Verification items for the finished model (mm, model axes). A direction names the side the tool comes from. Coordinates: 2 decimals unless noted, no trailing zeros. Loops run counter-clockwise (first coordinate to the right, second up) from the corner with the lowest first, then second, coordinate; pieces in that order, holes last. Notation, with made-up numbers: (-30, -20) -> (15, -20) arc R21 cw to (15, 7) -> close; hole circle Ø8 at (-28.5, -22.75). An arc over 180 degrees is marked (long way). Answer as a JSON object with one key per item and string values. Group by question number.
Q1. Scan lines: L1, parallel to X at y = 15, z = 50; L2, parallel to X at y = 47, z = 15; L3, parallel to Z at x = 48, y = 44. Record each from-to range of solid material in increasing order.
Q2. Cross-section at C-C on x = 21. Record the boundary of the cut face in (y, z), and give its area (3 significant figures).
Q3. Gauge pin test, flat ends, axial feed: pin 1 Ø10 at (x, z) = (52, 52) entering from +Y; pin 2 Ø10 at (x, y) = (47.5, 46.5) entering from +Z; pin 3 Ø1 at (y, z) = (49, 13) entering from -X. Record the tip position at first contact, or that the pin passes through.
Q4. Set-up check for faces 1 (the flat face through (50, 50, 40)), 2 (the flat face through (10, 10, 20)), 3 (the flat face through (60, 30, 30)), 4 (the flat face through (40, 40, 24)): record each of +Z, -Z, +X, -X, +Y, -Y from which the full face is reachable in a straight line by a thin tool's end or side.
Q5. Cross-section at D-D on y = 55. Record the boundary of the cut face in (x, z).
Q6. Cross-section at A-A on z = 35.5. Record the boundary of the cut face in (x, y).
Q7. Cross-section at B-B on y = 5. Record the boundary of the cut face in (x, z).
```python
from build123d import *

# Parameters (mm, degrees)
ESBO_O1_W                = 60
ESBO_O1_H                = 20
RESSALTO_EXTRUS_O1_DEPTH = 20
ESBO_O2_W                = 40
ESBO_O2_H                = 20
RESSALTO_EXTRUS_O2_DEPTH = 40
ESBO_O3_W                = 20
ESBO_O3_H                = 60
RESSALTO_EXTRUS_O3_DEPTH = 20
ESBO_O4_W                = 20
ESBO_O4_H                = 40
RESSALTO_EXTRUS_O4_DEPTH = 20


with BuildPart() as part:
    # Esboço1 → Ressalto-extrusão1 (new body)
    with BuildSketch(Plane.XY):
        with Locations((30, 10)):
            Rectangle(ESBO_O1_W, ESBO_O1_H)
    extrude(amount=RESSALTO_EXTRUS_O1_DEPTH)

    # Esboço2 → Ressalto-extrusão2 (add)
    with BuildSketch(Plane.XY.offset(20)):
        with Locations((40, 10)):
            Rectangle(ESBO_O2_W, ESBO_O2_H)
    extrude(amount=RESSALTO_EXTRUS_O2_DEPTH)

    # Esboço3 → Ressalto-extrusão3 (add)
    with BuildSketch(Plane(origin=(0, 20, 0), x_dir=(1, 0, 0), z_dir=(0, 1, 0))):
        with Locations((50, -30)):
            Rectangle(ESBO_O3_W, ESBO_O3_H)
    extrude(amount=RESSALTO_EXTRUS_O3_DEPTH)

    # Esboço4 → Ressalto-extrusão4 (add)
    with BuildSketch(Plane(origin=(0, 40, 0), x_dir=(1, 0, 0), z_dir=(0, 1, 0))):
        with Locations((50, -20)):
            Rectangle(ESBO_O4_W, ESBO_O4_H)
    extrude(amount=RESSALTO_EXTRUS_O4_DEPTH)


solid = part.part
```
Computed values:
{
 "1": {"L1": "x = 20 to 60", "L2": "x = 40 to 60", "L3": "z = 0 to 40"},
 "2": {"outline": "(0, 0) -> (20, 0) -> (20, 60) -> (0, 60) -> close", "area": "1,200 mm²"},
 "3": {"pin 1": "stops at y = 40", "pin 2": "stops at z = 40", "pin 3": "stops at x = 40"},
 "4": {"face 1": "+Z, +X, -X, +Y", "face 2": "+Z, -X, +Y, -Y", "face 3": "+Z, -Z, +X, +Y, -Y", "face 4": "+Z, -Z, -X, +Y"},
 "5": {"outline": "(40, 0) -> (60, 0) -> (60, 40) -> (40, 40) -> close"},
 "6": {"outline": "(20, 0) -> (60, 0) -> (60, 60) -> (40, 60) -> (40, 20) -> (20, 20) -> close"},
 "7": {"outline": "(0, 0) -> (60, 0) -> (60, 60) -> (20, 60) -> (20, 20) -> (0, 20) -> close"}
}
